Input: part model. Units: mm. Frame: model coordinates. A direction names the side the tool comes from. Round coordinates to 2 decimals unless told otherwise and drop trailing zeros. Order: outer loops, then holes, each group sorted by start corner. A loop starts at its lowest first (then second) coordinate and runs counter-clockwise, first axis right, second up. Notation, with made-up numbers: M -19,80 L 26,80 A20 ccw 26,107 Z; hole C 1,42 d7. An arc over 180 degrees is marked long. One line per question, with ' | ' between items.
```python
from build123d import *


with BuildPart() as part:
    # 草图2 → 旋转1 (revolve)
    with BuildSketch(Plane(origin=(0, 0, 0), x_dir=(0, 0, -1), z_dir=(1, 0, 0)), mode=Mode.PRIVATE) as revolve_1_sk:
        Polygon((0, 12.5), (50, 12.5), (50, 120.75), (46.446900937, 120.75), (44.081734967, 113.881059263), (35.918265033, 113.881059263), (33.553099063, 120.75), (31.446900937, 120.75), (29.081734967, 113.881059263), (20.918265033, 113.881059263), (18.553099063, 120.75), (16.446900937, 120.75), (14.081734967, 113.881059263), (5.918265033, 113.881059263), (3.553099063, 120.75), (0, 120.75), align=None)
    revolve(revolve_1_sk.sketch.rotate(Axis((0, 0, 0), (0, 0, -1)), 90), axis=Axis((0, 0, 0), (0, 0, -1)))


solid = part.part
```
Item 1: Access query for faces 4 (the cylindrical face through (108.62, -34.21, -39.94)), 5 (the flat face through (2, 25, -50)). Directions: +Z, -Z, +X, -X, +Y, -Y. A direction counts if a zero-diameter tool reaches every point of the face in a straight line with its end or side. Return the directions, or none.
Report:
face 4: none | face 5: -Z, +X, -X, +Y, -Y
Item 2: Line query: line 1 along Y through (x, z) = (0, -21); line 2 along Z through (x, y) = (-65, 99); line 3 along Z through (x, y) = (-74.5, -90). Output: solid intervals per line, ascending. Write a range as from..to.
Report:
line 1: -113.88..-12.5, 12.5..113.88 | line 2: -50..-45.65, -34.35..-30.65, -19.35..-15.65, -4.35..0 | line 3: -50..-45.1, -34.9..-30.1, -19.9..-15.1, -4.9..0
Item 3: Mould query, pull axis Y, two halves, no side actions, for faces 1 (the flat face through (-2, 25, 0)), 2 (the cylindrical face through (11.923, -3.755, -25.35)), 3 (the cylindrical face through (-26.176, 117.879, -48.199)). Classes: +Y half, -Y half, draft (parallel to the pull), parting line (faces both ways), or undercut.
Report:
face 1: draft | face 2: undercut | face 3: parting line
Item 4: Section query C-C, the plane z = -39.5. Return loops of the section in (x, y).
Report:
outline: C 0,0 d227.76; hole C 0,0 d25
Item 5: First-contact query: pin 1 (3 mm diameter, centred on x = -20.5, z = -40, fed in from +Y); pin 2 (10 mm diameter, centred on y = 14.5, z = -32, fed in from -X); pin 3 (8 mm diameter, centred on y = 46, z = -14.5, fed in from +X); pin 4 (20 mm diameter, centred on x = 0, y = 0, fed in from -Z). Flat tips, straight axial feed; report the tip coordinate or a pass-through.
Report:
pin 1: y = 112.28 | pin 2: x = -120.38 | pin 3: x = 113.02 | pin 4: through
